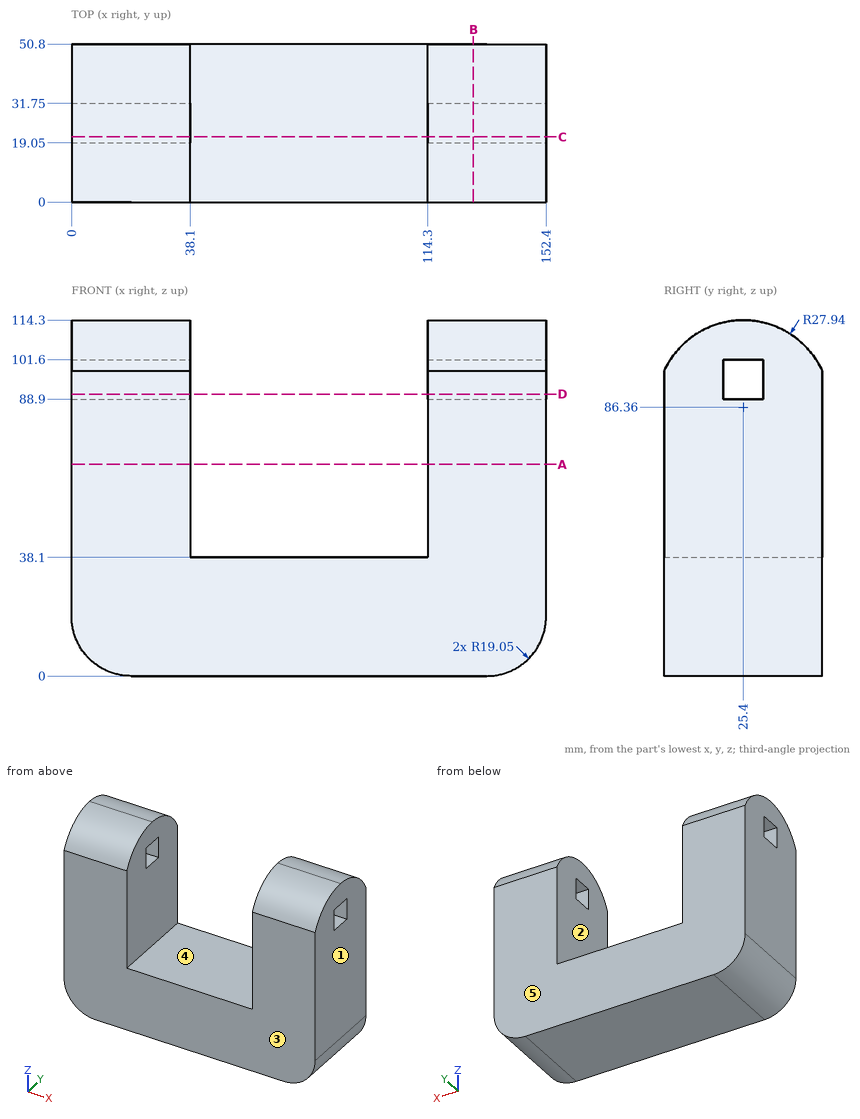
For this review, use the dimensioned drawing (mm, ordinates from the lowest corner) and the shaded views. A direction names the side the tool comes from. Give positions to 0.01 mm unless a question says otherwise; leave off trailing zeros. Loops run counter-clockwise (first coordinate to the right, second up) from the corner with the lowest first, then second, coordinate; pieces in that order, holes last.
Item 1: Take a section at A-A, the plane z = 68. State the section outline as (x, y) points.
Item 2: Tool access review of the marked faces 4 and 5: name each direction out of +Z, -Z, +X, -X, +Y, -Y from which nothing blocks a thin tool from reaching the whole face with its end or side.
Item 3: Take a section at C-C, the plane y = 21. State the section outline as (x, z) points, and give its area (3 significant figures).
Item 4: Take a section at B-B, the plane x = 129. State the section outline as (y, z) points.
Item 5: Draft analysis for pull direction X (two halves, no side actions). For the marked faces 1, 2 and 3, state which applies: +X half, -X half, draft (parallel to the pull), parting line (faces both ways), or undercut.
Item 6: For line 1 along X through (y, z) = (34, 41); line 2 along Z through (x, y) = (135.5, 31); line 3 along Z through (x, y) = (86, 11.5), list the stretches that pass through material, from the lowest coordinate up.
Item 7: Take a section at D-D, the plane z = 90.5. State the section outline as (x, y) points.
Item 8: Insertion check: pin 1 (4 mm diameter, centred on x = 10, y = 22.5, fed in from +Z); pin 2 (5 mm diameter, centred on x = 94, y = 35, fed in from +Z); pin 3 (3 mm diameter, centred on y = 15.5, z = 12.5, fed in from -X). Each pin has a flat end and moves straight along its axis. Give the tip position at first contact, or say it passes through.
Calculated:
1. outline: (0, 0) - (38.1, 0) - (38.1, 50.8) - (0, 50.8) - close; (114.3, 0) - (152.4, 0) - (152.4, 50.8) - (114.3, 50.8) - close
2. face 4: +Z, +Y, -Y
2. face 5: +Z, -Z, +X, -X, +Y
3. outline: (0, 19.05) arc R19.05 ccw to (19.05, 0) - (133.35, 0) arc R19.05 ccw to (152.4, 19.05) - (152.4, 88.9) - (114.3, 88.9) - (114.3, 38.1) - (38.1, 38.1) - (38.1, 88.9) - (0, 88.9) - close; (0, 101.6) - (38.1, 101.6) - (38.1, 113.95) - (0, 113.95) - close; (114.3, 101.6) - (152.4, 101.6) - (152.4, 113.95) - (114.3, 113.95) - close
3. area: 10,500 mm2
4. outline: (0, 0) - (50.8, 0) - (50.8, 98) arc R27.94 ccw to (25.4, 114.3) arc R27.94 ccw to (0, 98) - close; hole (19.05, 88.9) - (31.75, 88.9) - (31.75, 101.6) - (19.05, 101.6) - close
5. face 1: +X half
5. face 2: undercut
5. face 3: draft
6. line 1: x = 0 to 38.1, 114.3 to 152.4
6. line 2: z = 0.12 to 88.9, 101.6 to 113.73
6. line 3: z = 0 to 38.1
7. outline: (0, 0) - (38.1, 0) - (38.1, 19.05) - (0, 19.05) - close; (0, 31.75) - (38.1, 31.75) - (38.1, 50.8) - (0, 50.8) - close; (114.3, 0) - (152.4, 0) - (152.4, 19.05) - (114.3, 19.05) - close; (114.3, 31.75) - (152.4, 31.75) - (152.4, 50.8) - (114.3, 50.8) - close
8. pin 1: stops at z = 114.29
8. pin 2: stops at z = 38.1
8. pin 3: stops at x = 0.68
